from build123d import *

# Parameters (mm, degrees)
SKETCH_1_W          = 20
SKETCH_1_H          = 40
EXTRUDE_1_DEPTH     = 5
SKETCH_2_W          = 20
SKETCH_2_H          = 20
EXTRUDE_2_DEPTH     = 20
SKETCH_3_R          = 4.15
CUT_EXTRUDE_1_DEPTH = 42.044142746
FILLET_1_R          = 10
SKETCH_6_W          = 20
SKETCH_6_H          = 25.791536141
CUT_EXTRUDE_3_DEPTH = 54.65112416
SKETCH_7_W          = 20
SKETCH_7_H          = 5
EXTRUDE_5_DEPTH     = 10
SKETCH_8_W          = 20
SKETCH_8_H          = 5
EXTRUDE_6_DEPTH     = 10
SKETCH_10_R         = 1.6
CUT_EXTRUDE_5_DEPTH = 45.828803841
SKETCH_11_W         = 20
SKETCH_11_H         = 5
EXTRUDE_7_DEPTH     = 20
SKETCH_12_R         = 2.6
CUT_EXTRUDE_7_DEPTH = 82.655934826


with BuildPart() as part:
    # 草图1 → 凸台-拉伸1 (new body)
    with BuildSketch(Plane(origin=(0, 0, 0), x_dir=(1, 0, 0), z_dir=(0, 1, 0))):
        with Locations((2.634146341, -28.154142811)):
            Rectangle(SKETCH_1_W, SKETCH_1_H)
    extrude(amount=EXTRUDE_1_DEPTH)

    # 草图2 → 凸台-拉伸2 (add)
    with BuildSketch(Plane(origin=(0, 5, 0), x_dir=(1, 0, 0), z_dir=(0, 1, 0))):
        with Locations((2.634146341, -28.154142811)):
            Rectangle(SKETCH_2_W, SKETCH_2_H)
    extrude(amount=EXTRUDE_2_DEPTH)

    # 草图3 → 切除-拉伸1 (cut, through all)
    with BuildSketch(Plane.XY.offset(38.154142811)):
        with Locations((2.634146341, 15)):
            Circle(SKETCH_3_R)
    extrude(amount=-CUT_EXTRUDE_1_DEPTH, mode=Mode.SUBTRACT)

    # 圆角1
    fillet_1_edges = [part.edges().sort_by_distance(p)[0] for p in [
        (12.634146341, 25, 28.154142811),
        (-7.365853659, 25, 28.154142811),
    ]]
    fillet(fillet_1_edges, radius=FILLET_1_R - 0.0001)  # a hair under: the kernel refuses the full size

    # 草图6 → 切除-拉伸3 (cut, through all)
    with BuildSketch(Plane(origin=(0, 5, 0), x_dir=(1, 0, 0), z_dir=(0, 1, 0))):
        with Locations((2.634146341, -5.25837474)):
            Rectangle(SKETCH_6_W, SKETCH_6_H)
    extrude(amount=-CUT_EXTRUDE_3_DEPTH, mode=Mode.SUBTRACT)

    # 草图7 → 凸台-拉伸5 (add)
    with BuildSketch(Plane.XZ):
        with Locations((2.634146341, 20.654142811)):
            Rectangle(SKETCH_7_W, SKETCH_7_H)
    extrude(amount=EXTRUDE_5_DEPTH)

    # 草图8 → 凸台-拉伸6 (add)
    with BuildSketch(Plane.XY.offset(48.154142811)):
        with Locations((2.634146341, 2.5)):
            Rectangle(SKETCH_8_W, SKETCH_8_H)
    extrude(amount=EXTRUDE_6_DEPTH)

    # 草图10 → 切除-拉伸5 (cut, through all)
    with BuildSketch(Plane.XY.offset(23.154142811)):
        with Locations((2.634146341, -5)):
            Circle(SKETCH_10_R)
    extrude(amount=-CUT_EXTRUDE_5_DEPTH, mode=Mode.SUBTRACT)

    # 草图11 → 凸台-拉伸7 (add)
    with BuildSketch(Plane.XY.offset(58.154142811)):
        with Locations((2.634146341, 2.5)):
            Rectangle(SKETCH_11_W, SKETCH_11_H)
    extrude(amount=EXTRUDE_7_DEPTH)

    # 草图12 → 切除-拉伸7 (cut, through all)
    with BuildSketch(Plane(origin=(0, 5, 0), x_dir=(1, 0, 0), z_dir=(0, 1, 0))):
        with Locations(Location((2.634146341, -46.221727325, 0), (0, 0, 270))):
            Circle(SKETCH_12_R)
        with Locations(Location((2.634146341, -72.110167443, 0), (0, 0, 270))):
            Circle(SKETCH_12_R)
    extrude(amount=-CUT_EXTRUDE_7_DEPTH, mode=Mode.SUBTRACT)


solid = part.part
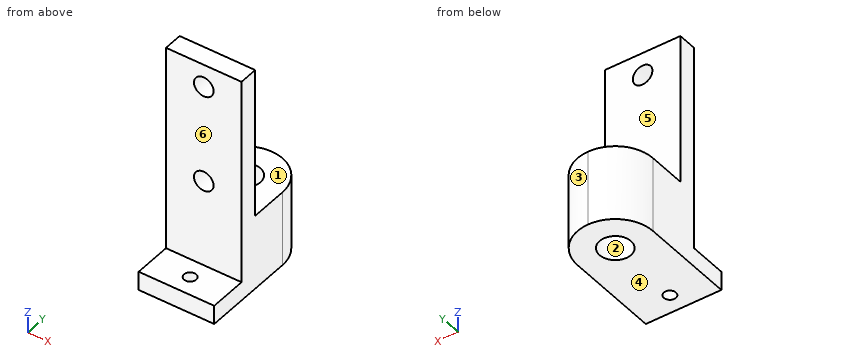
For this review, take the finished solid that the model builds, in its own axes (mm). Face numbers are marked on the shaded views. A direction names the side the tool comes from. Round coordinates to 2 decimals unless told otherwise and drop trailing zeros. Loops run counter-clockwise (first coordinate to the right, second up) from the corner with the lowest first, then second, coordinate; pieces in that order, holes last. Notation, with made-up numbers: (-12, 84) - (25, 84) arc R21 ccw to (25, 123) - close; hole circle Ø4 at (-9.5, 23.5). An arc over 180 degrees is marked (long way). One line per question, with ' | ' between items.
Q1. Take a section at A-A (y = -5). Give the boundary of the cut face in (x, z).
Taken from the geometry:
outline: (-7.37, 18.15) - (1.03, 18.15) - (1.03, 23.15) - (-7.37, 23.15) - close; (4.23, 18.15) - (12.63, 18.15) - (12.63, 23.15) - (4.23, 23.15) - close
Q2. For pin 1 (8 mm diameter, centred on x = 8, z = 48, fed in from -Y); pin 2 (6 mm diameter, centred on x = 7.5, z = 52.5, fed in from +Y); pin 3 (5 mm diameter, centred on x = -0.5, y = -7, fed in from +Z), all flat-tipped, find the tip position at first contact; note any pin that passes through.
Taken from the geometry:
pin 1: stops at y = 0 | pin 2: stops at y = 5 | pin 3: stops at z = 23.15
Q3. Tool access review of the marked faces 4, 5 and 6: name each direction out of +Z, -Z, +X, -X, +Y, -Y from which nothing blocks a thin tool from reaching the whole face with its end or side.
Taken from the geometry:
face 4: -Z, +X, -X, +Y, -Y | face 5: +Z, +X, -X, +Y | face 6: +Z, +X, -X, -Y
Q4. The part is to be moulded in two halves that separate along Y. For the marked faces 1, 2 and 3, say which applies: released by +Y, released by -Y, zero draft, split by the parting line, or undercut.
Taken from the geometry:
face 1: zero draft | face 2: undercut | face 3: released by +Y
Q5. Take a section at D-D (y = 6). Give the boundary of the cut face in (x, z).
Taken from the geometry:
outline: (-7.37, 18.15) - (12.63, 18.15) - (12.63, 38.15) - (-7.37, 38.15) - close
Q6. Take a section at B-B (z = 64). Give the boundary of the cut face in (x, y), and give its area (3 significant figures).
Taken from the geometry:
outline: (-7.37, 0) - (12.63, 0) - (12.63, 5) - (-7.37, 5) - close | area: 100 mm²
Q7. For line 1 along Y through (x, z) = (4.75, 62.5); line 2 along Z through (x, y) = (-2.25, 9); line 3 along Z through (x, y) = (-5.75, -1.5), list the stretches that pass through material, from the lowest coordinate up. Write a range as [from, to].
Taken from the geometry:
line 1: y = [0, 5] | line 2: z = [18.15, 38.15] | line 3: z = [18.15, 23.15]
Q8. Take a section at C-C (x = -3). Give the boundary of the cut face in (y, z), and give its area (3 significant figures).
Taken from the geometry:
outline: (-10, 18.15) - (23.26, 18.15) - (23.26, 38.15) - (5, 38.15) - (5, 78.15) - (0, 78.15) - (0, 23.15) - (-10, 23.15) - close | area: 715 mm²
